For this review, take the finished solid that the model builds, in its own axes (mm). A direction names the side the tool comes from. Coordinates: 2 decimals unless noted, no trailing zeros. Write each loop counter-clockwise with the first axis right and the second up, starting at its lowest first coordinate (ties: lowest second). Pieces come first, ordered by that corner, then holes. Notation, with made-up numbers: M 72.5,-16 L 83.5,-16 A11 ccw 83.5,-1 Z; hole C 62,73.5 d2. An arc over 180 degrees is marked long. Return JSON: item names as keys, results as strings.
```python
from build123d import *

# Parameters (mm, degrees)
F0_R     = 210.5
F1_DEPTH = 252
F2_R     = 183.5
F3_DEPTH = 231.775
F4_R     = 15
F5_R     = 5
F6_R     = 2


with BuildPart() as f1:
    # F0 (on Top) → F1 (new body)
    with BuildSketch(Plane.XY):
        Circle(F0_R)
    extrude(amount=F1_DEPTH)

    # F2 (on face) → F3 (cut)
    with BuildSketch(Plane.XY.offset(252)):
        Circle(F2_R)
    extrude(amount=-F3_DEPTH, mode=Mode.SUBTRACT)

    # F4
    f4_edges = [f1.edges().sort_by_distance(p)[0] for p in [
        (-210.5, 0, 0),
    ]]
    fillet(f4_edges, radius=F4_R)

    # F5
    f5_edges = [f1.edges().sort_by_distance(p)[0] for p in [
        (-210.5, 0, 252),
    ]]
    fillet(f5_edges, radius=F5_R)

    # F6
    f6_edges = [f1.edges().sort_by_distance(p)[0] for p in [
        (-183.5, 0, 252),
        (-183.5, 0, 20.225),
    ]]
    fillet(f6_edges, radius=F6_R)


solid = f1.part
```
1. For faces 1 (the face through (-31, 184, 252)), 2 (the face through (-3, 3, 20.225)), list the 3-axis set-ups (+Z, -Z, +X, -X, +Y, -Y) from which the entire face can be reached by the end or side of a thin tool; tool diameter is ignored.
Checks:
{"face 1": "+Z, +X, -X, +Y, -Y", "face 2": "+Z"}
2. Clearance check with flat-ended pins moving along their axes: pin 1 Ø12 at (x, y) = (91, 117.5) entering from +Z (3 decimals); pin 2 Ø1.5 at (y, z) = (-68, 185.5) entering from -X; pin 3 Ø12 at (y, z) = (48.5, 102) entering from +X (3 decimals). State where each tip first meets the part, or that it passes through.
Checks:
{"pin 1": "z = 20.225", "pin 2": "x = -199.47", "pin 3": "x = 206.165"}
3. Draft analysis for pull direction X (two halves, no side actions). For faces 3 (the face through (-23.89, 181.94, 137.71)), 4 (the face through (-3, 3, 0)), 5 (the face through (113.164, 177.494, 129.376)), state which applies: +X half, -X half, draft (parallel to the pull), parting line (faces both ways), or undercut.
Checks:
{"face 3": "undercut", "face 4": "draft", "face 5": "parting line"}
4. We need section C-C (z = 73). State the section outline as (x, y) points.
Checks:
{"outline": "C 0,0 d421; hole C 0,0 d367"}
5. We need section A-A (y = 0). State the section outline as (x, z) points (3 decimals), plus the area to 3 significant figures.
Checks:
{"outline": "M -210.5,15 A15 ccw -195.5,0 L 195.5,0 A15 ccw 210.5,15 L 210.5,247 A5 ccw 205.5,252 L 185.5,252 A2 ccw 183.5,250 L 183.5,22.225 A2 cw 181.5,20.225 L -181.5,20.225 A2 cw -183.5,22.225 L -183.5,250 A2 ccw -185.5,252 L -205.5,252 A5 ccw -210.5,247 Z", "area": "20,900 mm2"}
6. Wall thickness on L1, parallel to Y at x = 0, z = 179; L2, parallel to Z at x = -99.5, y = 108 (3 decimals); L3, parallel to X at y = 90, z = 201: over which ranges is each line inside the solid? List them lowest first. Write a range as from..to.
Checks:
{"L1": "-210.5..-183.5, 183.5..210.5", "L2": "0..20.225", "L3": "-190.29..-159.91, 159.91..190.29"}
